Part print with two shaded views. Sizes in mm from the minimum x, y, z corner. A direction names the side the tool comes from. Give positions to 0.01 mm unless a question says otherwise; leave off trailing zeros. Order: outer loops, then holes, each group sorted by start corner. A loop starts at its lowest first (then second) coordinate and runs counter-clockwise, first axis right, second up. Notation, with made-up numbers: (-25.75, 72) -> (30.25, 72) arc R37 ccw to (30.25, 109) -> close; hole circle Ø3 at (88.5, -27.5). An arc over 180 degrees is marked (long way). Write item = value, one per line. Start each with the question number.
Item 1: Pull direction X, two halves, no side cores. Call the marked faces 1, 2, 3 and 4: +X half, -X half, draft (parallel to the pull), parting line (faces both ways), or undercut.
Item 2: Band-saw the part on D-D on x = 10. Write the cut outline in (y, z).
Item 3: Band-saw the part on C-C on y = 8.75. Write the cut outline in (x, z), plus the area to 3 significant figures.
Item 4: Flat gauge pins, fed straight in: P1, Ø2, axis at x = 28.5, y = 8.5, coming from the -Z side; P2, Ø3, axis at y = 7.5, z = 30.5, coming from the +X side. Where does each tip first touch, or does it go through?
Item 5: Tool access for the marked faces 5 and 6: list every direction of +Z, -Z, +X, -X, +Y, -Y with a clear straight run to the whole face (end or side of a thin tool).
Item 6: Drill centre lines: line 1 along X through (y, z) = (8, 2); line 2 along X through (y, z) = (4.5, 10); line 3 along X through (y, z) = (5.5, 24). Where is each one in solid material? Low to high.
Item 7: Band-saw the part on A-A on z = 8. Write the cut outline in (x, y), plus the area to 3 significant figures.
Item 8: Band-saw the part on B-B on z = 28.5. Write the cut outline in (x, y).
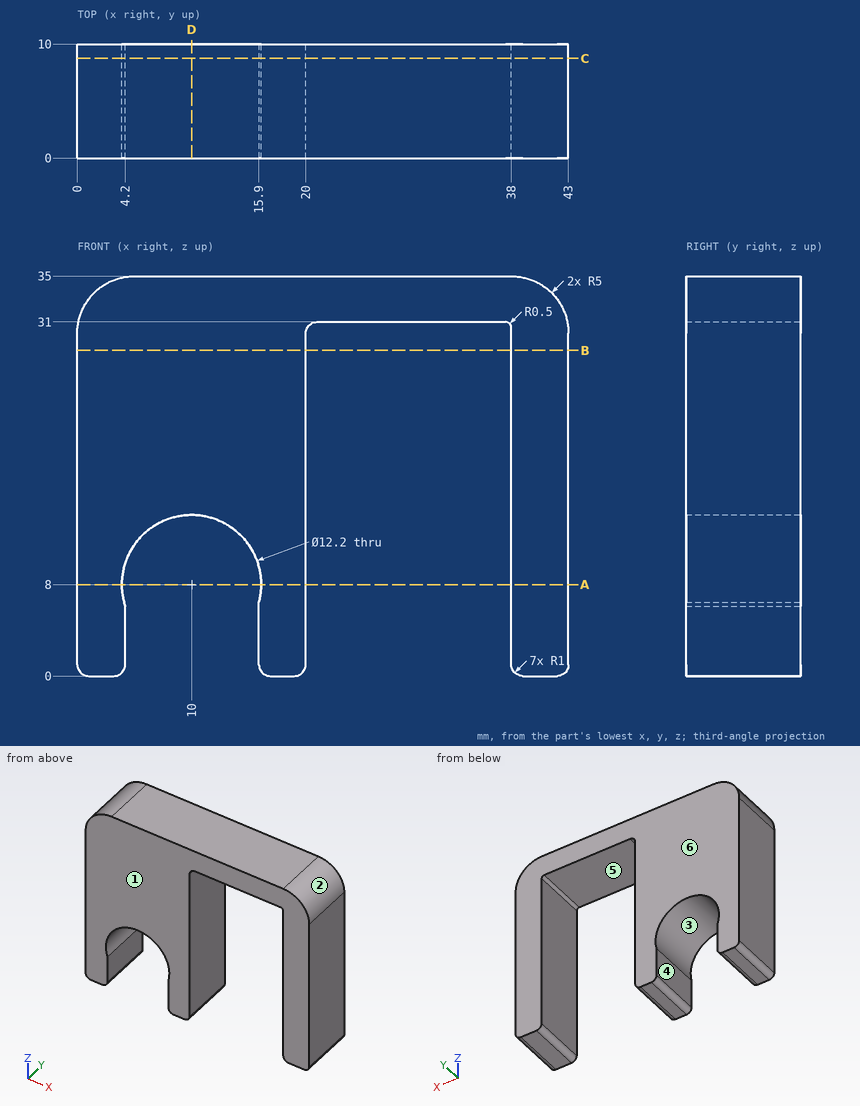
Values found:
q1.face_1 = draft
q1.face_2 = +X half
q1.face_3 = undercut
q1.face_4 = undercut
q2.outline = (0, 14.1) -> (10, 14.1) -> (10, 35) -> (0, 35) -> close
q3.outline = (0, 1) arc R1 ccw to (1, 0) -> (3.2, 0) arc R1 ccw to (4.2, 1) -> (4.2, 6.11) arc R6.1 cw (long way) to (15.9, 6.45) -> (15.9, 1) arc R1 ccw to (16.9, 0) -> (19, 0) arc R1 ccw to (20, 1) -> (20, 30) arc R1 cw to (21, 31) -> (37.5, 31) arc R0.5 cw to (38, 30.5) -> (38, 1) arc R1 ccw to (39, 0) -> (42, 0) arc R1 ccw to (43, 1) -> (43, 30) arc R5 ccw to (38, 35) -> (5, 35) arc R5 ccw to (0, 30) -> close
q3.area = 783 mm^2
q4.P1 = 31
q4.P2 = 43
q5.face_5 = -Z, +Y, -Y
q5.face_6 = +Z, -Z, +X, -X, +Y
q6.line_1 = 0 to 4.2, 15.9 to 20, 38 to 43
q6.line_2 = 0 to 4.24, 15.76 to 20, 38 to 43
q6.line_3 = 0 to 20, 38 to 43
q7.outline = (0, 0) -> (3.9, 0) -> (3.9, 10) -> (0, 10) -> close; (16.1, 0) -> (20, 0) -> (20, 10) -> (16.1, 10) -> close; (38, 0) -> (43, 0) -> (43, 10) -> (38, 10) -> close
q7.area = 128 mm^2
q8.outline = (0, 0) -> (20, 0) -> (20, 10) -> (0, 10) -> close; (38, 0) -> (43, 0) -> (43, 10) -> (38, 10) -> close
